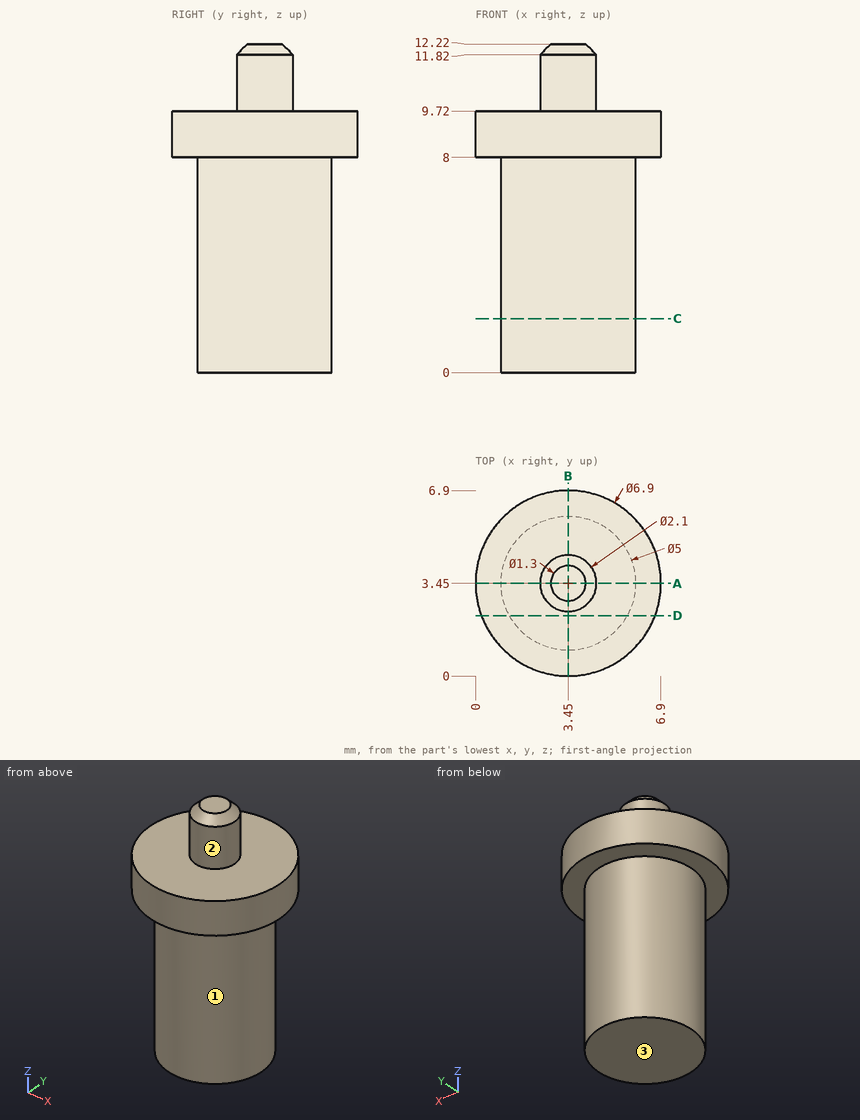
Source: three-view drawing plus pictorial views. Frame: mm from the lowest corner of the part. A direction names the side the tool comes from. Coordinates: 2 decimals unless noted, no trailing zeros. Order: outer loops, then holes, each group sorted by start corner. A loop starts at its lowest first (then second) coordinate and runs counter-clockwise, first axis right, second up.
Item 1: Cut plane C-C (z = 2). Return loops of the section in (x, y).
Output values:
outline: circle Ø5 at (3.45, 3.45)
Item 2: Set-up query: the marked faces 1, 2 and 3. Return all of +Z, -Z, +X, -X, +Y, -Y with unobstructed straight access to the full face (end or side cutting, diameter ignored); none if empty.
Output values:
face 1: -Z
face 2: +Z
face 3: -Z, +X, -X, +Y, -Y
Item 3: Cut plane D-D (y = 2.25). Return loops of the section in (x, z), plus the area to 3 significant figures.
Output values:
outline: (0.22, 8) - (1.26, 8) - (1.26, 0) - (5.64, 0) - (5.64, 8) - (6.68, 8) - (6.68, 9.72) - (0.22, 9.72) - close
area: 46.2 mm2
Item 4: First-contact query: P1, Ø4, axis at y = 4, z = 4.5, coming from the -X side; P2, Ø1, axis at x = 4.5, y = 0.5, coming from the +Z side; P3, Ø1, axis at y = 1.5, z = 10, coming from the -X side. Flat tips, straight axial feed; report the tip coordinate or a pass-through.
Output values:
P1: stops at x = 0.95
P2: stops at z = 9.72
P3: stops at x = 0.36
Item 5: Material intervals for line 1 (Z direction, x = 5.75, y = 4); line 2 (Z direction, x = 1.5, y = 5.75); line 3 (Y direction, x = 4.5, z = 3.5), sorted ascending.
Output values:
line 1: z = 0 to 9.72
line 2: z = 8 to 9.72
line 3: y = 1.18 to 5.72
Item 6: Cut plane A-A (y = 3.45). Return loops of the section in (x, z).
Output values:
outline: (0, 8) - (0.95, 8) - (0.95, 0) - (5.95, 0) - (5.95, 8) - (6.9, 8) - (6.9, 9.72) - (4.5, 9.72) - (4.5, 11.82) - (4.1, 12.22) - (2.8, 12.22) - (2.4, 11.82) - (2.4, 9.72) - (0, 9.72) - close
